Here's how the part is built. I have some questions about the finished solid (model axes, mm). Coordinates: 2 decimals unless noted, no trailing zeros. Write each loop counter-clockwise with the first axis right and the second up, starting at its lowest first coordinate (ties: lowest second). Pieces come first, ordered by that corner, then holes.
Item 1: I want a section at C-C (y = -34.6). Please give me the cut outline in (x, z), and give its area (3 significant figures).
Item 2: I'm going to push a flat-ended pin straight in: P1, Ø12, axis at x = -41, z = -0.5, coming from the +Y side. Where does the tip first touch, or does it pass through?
Item 3: I want a section at B-B (x = 8.5). Please give me the cut outline in (y, z), and give its area (3 significant figures).
Item 4: I want a section at A-A (z = -4). Please give me the cut outline in (x, y).
Item 5: Please list where these lines run through material, in increasing order: line 1 (Z direction, x = -35, y = -34.55); line 2 (X direction, y = -34.55, z = -17).
from build123d import *

# Parameters (mm, degrees)
SKETCH1_W           = 126
SKETCH1_H           = 66
SKETCH1_W_2         = 84.5
SKETCH1_H_2         = 57
BOSS_EXTRUDE1_DEPTH = 0.3
FILLET1_R           = 2


with BuildPart() as part:
    # Sketch1 → Boss-Extrude1 (new body)
    with BuildSketch(Plane.XZ.offset(34.5)):
        Rectangle(SKETCH1_W, SKETCH1_H)
        Rectangle(SKETCH1_W_2, SKETCH1_H_2, mode=Mode.SUBTRACT)
    extrude(amount=BOSS_EXTRUDE1_DEPTH)

    # Fillet1
    fillet1_edges = [part.edges().sort_by_distance(p)[0] for p in [
        (63, -34.65, -33),
        (-63, -34.65, -33),
        (-63, -34.65, 33),
        (63, -34.65, 33),
    ]]
    fillet(fillet1_edges, radius=FILLET1_R)


solid = part.part
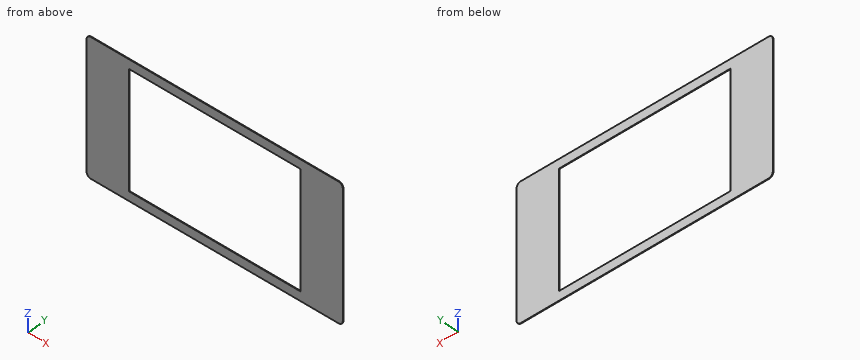
Answer:
1. outline: (-63, -31) arc R2 ccw to (-61, -33) - (61, -33) arc R2 ccw to (63, -31) - (63, 31) arc R2 ccw to (61, 33) - (-61, 33) arc R2 ccw to (-63, 31) - close; hole (-42.25, -28.5) - (42.25, -28.5) - (42.25, 28.5) - (-42.25, 28.5) - close
1. area: 3,500 mm2
2. P1: stops at y = -34.5
3. outline: (-34.8, -33) - (-34.5, -33) - (-34.5, -28.5) - (-34.8, -28.5) - close; (-34.8, 28.5) - (-34.5, 28.5) - (-34.5, 33) - (-34.8, 33) - close
3. area: 2.70 mm2
4. outline: (-63, -34.8) - (-42.25, -34.8) - (-42.25, -34.5) - (-63, -34.5) - close; (42.25, -34.8) - (63, -34.8) - (63, -34.5) - (42.25, -34.5) - close
5. line 1: z = -33 to -28.5, 28.5 to 33
5. line 2: x = -63 to -42.25, 42.25 to 63
